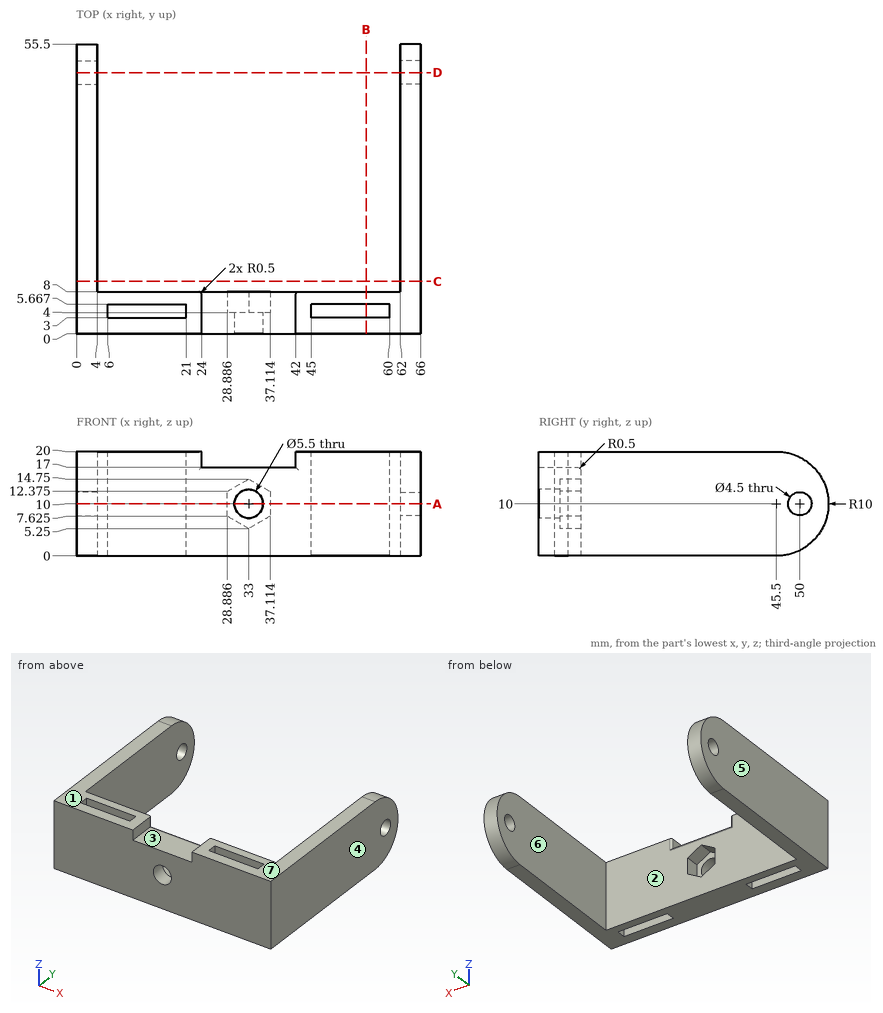
For this review, use the dimensioned drawing (mm, ordinates from the lowest corner) and the shaded views. A direction names the side the tool comes from. Round coordinates to 2 decimals unless told otherwise and drop trailing zeros. Write each loop counter-clockwise with the first axis right and the second up, starting at its lowest first coordinate (ties: lowest second). Pieces come first, ordered by that corner, then holes. Notation, with made-up numbers: (7.25, -38.75) -> (56.25, -38.75) arc R28 ccw to (56.25, -17.75) -> close; hole circle Ø6 at (39, -8.5). An arc over 180 degrees is marked (long way). One line per item, written item: value. Start each with the question number.
Q1. Insertion check: P1, Ø6, axis at x = 41.5, z = 13, coming from the +Y side; P2, Ø6, axis at x = 34.5, y = 4, coming from the +Z side. Each pin has a flat end and moves straight along its axis. Give the tip position at first contact, or say it passes through.
Q2. The part is to be moulded in two halves that separate along X. For the marked faces 4, 5, 6 and 7, say which applies: pulls with the +X half, pulls with the -X half, needs draft (parallel to the pull), parting line crosses it, or undercut.
Q3. Tool access review of the marked faces 1, 2 and 3: name each direction out of +Z, -Z, +X, -X, +Y, -Y from which nothing blocks a thin tool from reaching the whole face with its end or side.
Q4. To check wall thickness, follow probe 1 along Y at (x, z) = (7, 13.5); probe 2 along X at (y, z) = (20, 5.25); probe 3 along Z at (x, y) = (33, 2). State the ranges of each line that lie inside material, in increasing order.
Q5. Add section D-D (y = 50). Give the boundary of the cut face in (x, z).
Q6. Add section B-B (x = 55.5). Give the boundary of the cut face in (y, z).
Q7. Add section C-C (y = 10). Give the boundary of the cut face in (x, z).
Q8. Add section A-A (z = 10). State how many separate pieces and enclosed holes the cut face has, then the cut area to 3 significant figures.
Response:
1. P1: stops at y = 8
1. P2: stops at z = 17
2. face 4: pulls with the +X half
2. face 5: pulls with the -X half
2. face 6: undercut
2. face 7: needs draft
3. face 1: +Z, +X, -X, +Y, -Y
3. face 2: +Z, -Z, +Y
3. face 3: +Z, +Y, -Y
4. probe 1: y = 0 to 3, 5.67 to 8
4. probe 2: x = 0 to 4, 62 to 66
4. probe 3: z = 0 to 7.25, 12.75 to 17
5. outline: (0, 1.07) -> (4, 1.07) -> (4, 7.75) -> (0, 7.75) -> close; (0, 12.25) -> (4, 12.25) -> (4, 18.93) -> (0, 18.93) -> close; (62, 1.07) -> (66, 1.07) -> (66, 7.75) -> (62, 7.75) -> close; (62, 12.25) -> (66, 12.25) -> (66, 18.93) -> (62, 18.93) -> close
6. outline: (0, 0) -> (3, 0) -> (3, 20) -> (0, 20) -> close; (5.67, 0) -> (8, 0) -> (8, 20) -> (5.67, 20) -> close
7. outline: (0, 0) -> (4, 0) -> (4, 20) -> (0, 20) -> close; (62, 0) -> (66, 0) -> (66, 20) -> (62, 20) -> close
8. separate pieces: 4
8. enclosed holes: 2
8. area: 737 mm^2
